Work out the finished part from the listing and answer in its coordinate system (mm). A direction names the side the tool comes from. Give positions to 0.01 mm unless a question says otherwise; leave off trailing zeros. Loops run counter-clockwise (first coordinate to the right, second up) from the corner with the lowest first, then second, coordinate; pieces in that order, holes last. Notation, with made-up numbers: (-6.5, 64) - (7.5, 64) arc R17 ccw to (7.5, 72) - close; hole circle Ø1 at (81.25, 61.5). An arc over 180 degrees is marked (long way). One line per item, written item: value.
from build123d import *

# Parameters (mm, degrees)
SKETCH1_W               = 24
SKETCH1_H               = 24
BOSS_EXTRUDE1_DEPTH     = 100
SKETCH2_R               = 9
CUT_EXTRUDE1_DEPTH      = 100
SKETCH3_W               = 24
SKETCH3_H               = 24
BOSS_EXTRUDE2_DEPTH     = 50
SKETCH4_R               = 9
CUT_EXTRUDE2_DEPTH      = 50
SKETCH5_R               = 3
BOSS_EXTRUDE3_DEPTH     = 24
SKETCH6_R               = 1.5
CUT_EXTRUDE3_DEPTH      = 24
CUT_EXTRUDE4_DEPTH      = 115.350338871
CUT_EXTRUDE4_DEPTH_BACK = 115.350338871
SKETCH7_W               = 77
SKETCH7_H               = 15


with BuildPart() as part:
    # Sketch1 → Boss-Extrude1 (new body)
    with BuildSketch(Plane(origin=(0, 0, 0), x_dir=(0, 0, -1), z_dir=(1, 0, 0))):
        with Locations((12, 12)):
            Rectangle(SKETCH1_W, SKETCH1_H)
    extrude(amount=BOSS_EXTRUDE1_DEPTH)

    # Sketch2 → Cut-Extrude1 (cut)
    with BuildSketch(Plane(origin=(100, 0, 0), x_dir=(0, 0, -1), z_dir=(1, 0, 0))):
        with Locations((12, 12)):
            Circle(SKETCH2_R)
    extrude(amount=-CUT_EXTRUDE1_DEPTH, mode=Mode.SUBTRACT)

    # Sketch3 → Boss-Extrude2 (add)
    with BuildSketch(Plane.XY):
        with Locations((27, 12)):
            Rectangle(SKETCH3_W, SKETCH3_H)
    extrude(amount=BOSS_EXTRUDE2_DEPTH)

    # Sketch4 → Cut-Extrude2 (cut)
    with BuildSketch(Plane.XY.offset(50)):
        with Locations((27, 12)):
            Circle(SKETCH4_R)
    extrude(amount=-CUT_EXTRUDE2_DEPTH, mode=Mode.SUBTRACT)

    # Sketch5 → Boss-Extrude3 (add)
    with BuildSketch(Plane(origin=(0, 24, 0), x_dir=(1, 0, 0), z_dir=(0, 1, 0))):
        with Locations((90, 0)):
            Circle(SKETCH5_R)
        with Locations((90, 24)):
            Circle(SKETCH5_R)
        with Locations((50, 0)):
            Circle(SKETCH5_R)
        with Locations((50, 24)):
            Circle(SKETCH5_R)
        with Locations((7.5, 0)):
            Circle(SKETCH5_R)
        with Locations((7.5, 24)):
            Circle(SKETCH5_R)
        with Locations((15, -10)):
            Circle(SKETCH5_R)
        with Locations((39, -10)):
            Circle(SKETCH5_R)
        with Locations((15, -40)):
            Circle(SKETCH5_R)
        with Locations((39, -40)):
            Circle(SKETCH5_R)
    extrude(amount=-BOSS_EXTRUDE3_DEPTH)

    # Sketch6 → Cut-Extrude3 (cut)
    with BuildSketch(Plane(origin=(0, 24, 0), x_dir=(1, 0, 0), z_dir=(0, 1, 0))):
        with Locations(Location((50, 24, 0), (0, 0, 270))):
            Circle(SKETCH6_R)
        with Locations(Location((50, 0, 0), (0, 0, 270))):
            Circle(SKETCH6_R)
        with Locations(Location((90, 24, 0), (0, 0, 270))):
            Circle(SKETCH6_R)
        with Locations(Location((90, 0, 0), (0, 0, 270))):
            Circle(SKETCH6_R)
        with Locations(Location((15, -40, 0), (0, 0, 270))):
            Circle(SKETCH6_R)
        with Locations(Location((15, -10, 0), (0, 0, 270))):
            Circle(SKETCH6_R)
        with Locations(Location((39, -10, 0), (0, 0, 270))):
            Circle(SKETCH6_R)
        with Locations(Location((39, -40, 0), (0, 0, 270))):
            Circle(SKETCH6_R)
        with Locations(Location((7.5, 0, 0), (0, 0, 270))):
            Circle(SKETCH6_R)
        with Locations(Location((7.5, 24, 0), (0, 0, 270))):
            Circle(SKETCH6_R)
    extrude(amount=-CUT_EXTRUDE3_DEPTH, mode=Mode.SUBTRACT)

    # Sketch7 → Cut-Extrude4 (cut, two sides: drawn at the far end of the back side and taken through both)
    with BuildSketch(Plane(origin=(100, 0, 0), x_dir=(0, 0, -1), z_dir=(1, 0, 0)).offset(-CUT_EXTRUDE4_DEPTH_BACK)):
        with Locations((-11.5, 7.5)):
            Rectangle(SKETCH7_W, SKETCH7_H)
    extrude(amount=CUT_EXTRUDE4_DEPTH + CUT_EXTRUDE4_DEPTH_BACK, mode=Mode.SUBTRACT)


solid = part.part
1. Section B-B (x = 90) is taken. Write down the section's boundary in (y, z), and give its area (3 significant figures).
Output:
outline: (15, -27) - (24, -27) - (24, -25.5) - (15, -25.5) - close; (15, -22.5) - (24, -22.5) - (24, -1.5) - (15, -1.5) - (15, -3.51) arc R9 cw to (15, -20.49) - close; (15, 1.5) - (24, 1.5) - (24, 3) - (15, 3) - close
area: 142 mm²
2. Section A-A (z = 40) is taken. Write down the section's boundary in (x, y), and give its area (3 significant figures).
Output:
outline: (12, 15) - (13.5, 15) - (13.5, 24) - (12, 24) - close; (16.5, 15) - (18.51, 15) arc R9 cw to (35.49, 15) - (37.5, 15) - (37.5, 24) - (16.5, 24) - close; (40.5, 15) - (42, 15) - (42, 24) - (40.5, 24) - close
area: 142 mm²
3. The mould has two halves that part along X. Classify faces 5 (the cylindrical face through (48.536, 19.563, -24.325)), 6 (the flat face through (28, 19, -24)), 7 (the flat face through (38.7, 15, 13.5)), 8 (the cylindrical face through (12, 20, 40)): released by +X, released by -X, zero draft, split by the parting line, or undercut.
Output:
face 5: undercut
face 6: undercut
face 7: zero draft
face 8: released by -X
4. Section D-D (y = 16.75) is taken. Count the separate pieces of the cut face and the enclosed holes in it, and give its area (3 significant figures).
Output:
separate pieces: 2
enclosed holes: 10
area: 1,380 mm²
5. Section C-C (x = 67) is taken. Write down the section's boundary in (y, z).
Output:
outline: (15, -24) - (24, -24) - (24, 0) - (15, 0) - (15, -3.51) arc R9 cw to (15, -20.49) - close
6. Flat-ended cylindrical pins translate along their axes: pin 1 Ø1.3 at (x, y) = (2.5, 20) entering from +Z; pin 2 Ø1 at (y, z) = (18, 35.5) entering from +X; pin 3 Ø2.5 at (x, y) = (41.5, 21) entering from +Z. Find the tip coordinate at first contact, or state that the pin passes through.
Output:
pin 1: stops at z = 0
pin 2: stops at x = 39
pin 3: stops at z = 42.73
7. Find the intervals of material crossed by line 1 along X through (y, z) = (19.5, 10); line 2 along X through (y, z) = (22.5, 9.5); line 3 along X through (y, z) = (17.75, 10), in increasing order.
Output:
line 1: x = 12 to 13.5, 16.5 to 22.03, 31.97 to 37.5, 40.5 to 42
line 2: x = 12.04 to 13.59, 16.41 to 37.59, 40.41 to 41.96
line 3: x = 12 to 13.5, 16.5 to 20.08, 33.92 to 37.5, 40.5 to 42
8. For faces 1 (the flat face through (15, 19, 3)), 2 (the flat face through (70, 19, 0)), 3 (the flat face through (27, 17, 0)), 4 (the flat face through (96, 19, -24)), determine the directions among +Z, -Z, +X, -X, +Y, -Y from which every point of the face is accessible in a straight line to the end or side of a thin tool.
Output:
face 1: +Y, -Y
face 2: +Z, +Y, -Y
face 3: +Z, -Y
face 4: -Z, +X, +Y, -Y
